```python
from build123d import *

# Parameters (mm, degrees)
CROQUIS1_R              = 32.5
SALIENTE_EXTRUIR1_DEPTH = 19.5
VACIADO1_T              = -2.5
CROQUIS2_R              = 15
CORTAR_EXTRUIR1_DEPTH   = 19.5
SALIENTE_EXTRUIR2_DEPTH = 1.5
MATRIZC2_COUNT          = 4


with BuildPart() as part:
    # Croquis1 → Saliente-Extruir1 (new body)
    with BuildSketch(Plane(origin=(0, 0, 0), x_dir=(1, 0, 0), z_dir=(0, 1, 0))):
        with Locations(Location((0, 0, 0), (0, 0, 270))):
            Circle(CROQUIS1_R)
    extrude(amount=SALIENTE_EXTRUIR1_DEPTH)

    # Vaciado1
    vaciado1_openings = [part.faces().sort_by_distance(p)[0] for p in [
        (0, 0, 0),
    ]]
    offset(amount=VACIADO1_T, openings=vaciado1_openings, kind=Kind.INTERSECTION)

    # Croquis2 → Cortar-Extruir1 (cut)
    with BuildSketch(Plane(origin=(0, 19.5, 0), x_dir=(1, 0, 0), z_dir=(0, 1, 0))):
        with Locations(Location((0, 0, 0), (0, 0, 270))):
            Circle(CROQUIS2_R)
    extrude(amount=-CORTAR_EXTRUIR1_DEPTH, mode=Mode.SUBTRACT)

    # Croquis3 → Saliente-Extruir2 (add, symmetric)
    with BuildSketch(Plane(origin=(0, 0, 0), x_dir=(0, 0, -1), z_dir=(1, 0, 0))):
        Polygon((-30, 4), (-28.1, 4), (-28.1, 6), (-30, 8), align=None)
    saliente_extruir2 = extrude(amount=SALIENTE_EXTRUIR2_DEPTH, both=True)

    # MatrizC2: Saliente-Extruir2 ×4 about axis
    matrizc2_axis = Axis((0, 0, 0), (0, 1, 0))
    for i in range(1, MATRIZC2_COUNT):
        add(saliente_extruir2.rotate(matrizc2_axis, i * 360 / MATRIZC2_COUNT))


solid = part.part
```
For this review, take the finished solid that the model builds, in its own axes (mm). A direction names the side the tool comes from. Round coordinates to 2 decimals unless told otherwise and drop trailing zeros. Write each loop counter-clockwise with the first axis right and the second up, starting at its lowest first coordinate (ties: lowest second). Pieces come first, ordered by that corner, then holes. Notation, with made-up numbers: (72, 3) -> (106, 3) arc R20 ccw to (106, 37) -> close; hole circle Ø6 at (-8, 56). An arc over 180 degrees is marked (long way). One line per question, with ' | ' between items. Start each with the question number.
(1) For line 1 along X through (y, z) = (13, 0); line 2 along X through (y, z) = (5.5, 0); line 3 along Z through (x, y) = (11.5, 5.25), list the stretches that pass through material, from the lowest coordinate up. Write a range as from..to.
(2) Mouldability with a two-part tool opening along Z and no side actions: class faces 4 (the face through (0, 5, -28.1)), 5 (the face through (-7, 19.5, 14)), 6 (the face through (9.76, 9.61, 31)) as released by +Z, released by -Z, zero draft, split by the parting line, or undercut.
(3) Tool access review of faces 1 (the face through (-1.5, 6, 29)), 2 (the face through (-0.02, 6.99, -29.04)), 3 (the face through (0.66, 18.268, -14.985)): name each direction out of +Z, -Z, +X, -X, +Y, -Y from which nothing blocks a thin tool from reaching the whole face with its end or side.
(4) Add section D-D, the plane z = 18. Write out the cut boundary in (x, y).
(5) Add section B-B, the plane z = -3.5. Write out the cut boundary in (x, y), plus the area to 3 significant figures.
(6) Add section C-C, the plane y = 3. Write out the cut boundary in (x, z), plus the area to 3 significant figures.
(7) Insertion check: P1, Ø1.5, axis at x = 19.5, y = 7, coming from the +Z side; P2, Ø0.6, axis at x = 29, y = 6, coming from the +Z side; P3, Ø3, axis at x = 6, y = 16.5, coming from the -Z side. Each pin has a flat end and moves straight along its axis. Give the tip position at first contact, or say it passes through.
(8) Add section A-A, the plane x = 0. Write out the cut boundary in (y, z), plus the area to 3 significant figures.
Answer list:
1) line 1: -32.5..-30, 30..32.5 | line 2: -32.5..-28.1, 28.1..32.5 | line 3: -30.4..-27.71, 27.71..30.4
2) face 4: undercut | face 5: zero draft | face 6: split by the parting line
3) face 1: -Y | face 2: none | face 3: +Y, -Y
4) outline: (-27.06, 0) -> (-24, 0) -> (-24, 17) -> (24, 17) -> (24, 0) -> (27.06, 0) -> (27.06, 19.5) -> (-27.06, 19.5) -> close
5) outline: (-32.31, 0) -> (-29.8, 0) -> (-29.8, 17) -> (-14.59, 17) -> (-14.59, 19.5) -> (-32.31, 19.5) -> close; (14.59, 17) -> (29.8, 17) -> (29.8, 0) -> (32.31, 0) -> (32.31, 19.5) -> (14.59, 19.5) -> close | area: 174 mm²
6) outline: circle Ø65 at (0, 0); hole circle Ø60 at (0, 0) | area: 491 mm²
7) P1: z = 26.55 | P2: z = 15.25 | P3: z = -32.19
8) outline: (0, -32.5) -> (19.5, -32.5) -> (19.5, -15) -> (17, -15) -> (17, -30) -> (8, -30) -> (6, -28.1) -> (4, -28.1) -> (4, -30) -> (0, -30) -> close; (0, 30) -> (4, 30) -> (4, 28.1) -> (6, 28.1) -> (8, 30) -> (17, 30) -> (17, 15) -> (19.5, 15) -> (19.5, 32.5) -> (0, 32.5) -> close | area: 184 mm²
